Here's how the part is built. I have some questions about the finished solid (model axes, mm). Round coordinates to 2 decimals unless told otherwise and drop trailing zeros. Loops run counter-clockwise (first coordinate to the right, second up) from the corner with the lowest first, then second, coordinate; pieces in that order, holes last. Notation, with made-up numbers: (84, -30.5) -> (93, -30.5) arc R25 ccw to (93, 1.5) -> close; hole circle Ø6 at (77, 60). An arc over 180 degrees is marked (long way). Use one line per item in the form item = value. Start each with the question number.
Item 1: I'm going to push a flat-ended pin straight in: pin 1 Ø10 at (x, z) = (82, -82) entering from +Y. Where does the tip first touch, or does it pass through?
Item 2: If I drill on L1, parallel to X at y = 7.75, z = -82; L2, parallel to Z at x = 84, y = 6.25; L3, parallel to X at y = 1, z = -40, over which ranges is the centre line in solid material (lowest first)? Write a range as [from, to].
Item 3: If we section it at A-A (x = 82): Write out the boundary of the cut face in (y, z).
Item 4: If we section it at B-B (z = -82): Write out the boundary of the cut face in (x, y).
```python
from build123d import *

# Parameters (mm, degrees)
SKETCH1_W           = 220
SKETCH1_H           = 220
SKETCH1_W_2         = 194
SKETCH1_H_2         = 194
SKETCH1_R           = 8.5
BOSS_EXTRUDE1_DEPTH = 10
FILLET1_R           = 2
FILLET2_R           = 2


with BuildPart() as part:
    # Sketch1 → Boss-Extrude1 (new body)
    # profile 1 of 2: a face of its own
    with BuildSketch(Plane(origin=(0, 0, 0), x_dir=(1, 0, 0), z_dir=(0, 1, 0))):
        Rectangle(SKETCH1_W, SKETCH1_H)
        Rectangle(SKETCH1_W_2, SKETCH1_H_2, mode=Mode.SUBTRACT)
    # profile 2 of 2: a face of its own
    with BuildSketch(Plane(origin=(0, 0, 0), x_dir=(1, 0, 0), z_dir=(0, 1, 0))):
        Rectangle(SKETCH1_W_2, SKETCH1_H_2)
        with Locations(Location((82, 82, 0), (0, 0, 270))):
            Circle(SKETCH1_R, mode=Mode.SUBTRACT)
    extrude(amount=BOSS_EXTRUDE1_DEPTH)

    # Fillet1
    fillet1_edges = [part.edges().sort_by_distance(p)[0] for p in [
        (110, 5, 110),
        (-110, 5, 110),
        (-110, 5, -110),
        (110, 5, -110),
    ]]
    fillet(fillet1_edges, radius=FILLET1_R)

    # Fillet2
    fillet2_edges = [part.edges().sort_by_distance(p)[0] for p in [
        (0, 0, 110),
        (110, 0, 0),
        (-110, 0, 0),
        (0, 0, -110),
        (109.414213562, 0, 109.414213562),
        (109.414213562, 0, -109.414213562),
        (-109.414213562, 0, -109.414213562),
        (-109.414213562, 0, 109.414213562),
        (82, 0, -90.5),
    ]]
    fillet(fillet2_edges, radius=FILLET2_R)


solid = part.part
```
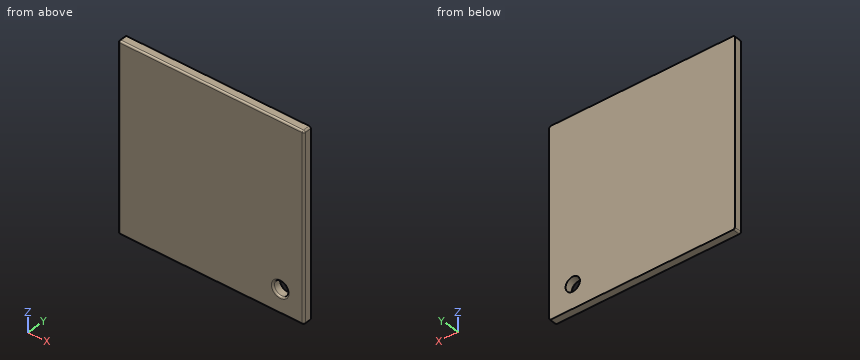
Values found:
q1.pin_1 = through
q2.L1 = [-110, 73.5], [90.5, 110]
q2.L2 = [-110, -90.26], [-73.74, 110]
q2.L3 = [-109.73, 109.73]
q3.outline = (0, -108) arc R2 ccw to (2, -110) -> (10, -110) -> (10, -90.5) -> (2, -90.5) arc R2 ccw to (0, -92.5) -> close; (0, -71.5) arc R2 ccw to (2, -73.5) -> (10, -73.5) -> (10, 110) -> (2, 110) arc R2 ccw to (0, 108) -> close
q4.outline = (-110, 2) arc R2 ccw to (-108, 0) -> (71.5, 0) arc R2 ccw to (73.5, 2) -> (73.5, 10) -> (-110, 10) -> close; (90.5, 2) arc R2 ccw to (92.5, 0) -> (108, 0) arc R2 ccw to (110, 2) -> (110, 10) -> (90.5, 10) -> close
